Can you work these out from the model? Positions are in its coordinate system, mm. A direction names the side the tool comes from. Give positions to 0.01 mm unless a question says otherwise; leave off trailing zeros. Order: outer loops, then holes, each group sorted by start corner. A loop starts at its lowest first (then second) coordinate and runs counter-clockwise, first axis right, second up. Notation, with made-up numbers: M 51.25,15.5 L 73.25,15.5 A10 cw 73.25,25.5 Z; hole C 80,-5 d4. An arc over 180 degrees is marked long. One line per question, with ' | ' between items. Start each with the question number.
1) Thinking about a two-plate mould opening in X: for faces 1 (the cylindrical face through (-2.343, 17.847, 0.182)), 2 (the cylindrical face through (0.1, -3.1, 0.2)), 3 (the flat face through (0, -4, 13)), which applies, +X half, -X half, draft (parallel to the pull), parting line (faces both ways), or undercut?
2) If we section it at C-C, the plane z = 7.25: Please give me the cut outline in (x, y).
3) If we section it at B-B, the plane x = 0: Please give me the cut outline in (y, z), plus the area to 3 significant figures.
4) If we section it at A-A, the plane y = 0: Please give me the cut outline in (x, z).
5) Please list where these lines run through material, in increasing order: line 1 along Y through (x, z) = (0, -7.5); line 2 along X through (y, z) = (3.5, -6.25); line 3 along X through (y, z) = (13, 0). Write a range as [from, to].
6) If we section it at D-D, the plane y = 14: Please give me the cut outline in (x, z).
7) For faces 4 (the flat face through (-1, 3.5, 0.2)), 5 (the flat face through (0, -4, -13)), which set-ups out of +Z, -Z, +X, -X, +Y, -Y let a thin tool reach every point of the face, with its end or its side?
8) I'm going to push flat-ended pins straight in: pin 1 Ø1.2 at (y, z) = (3.5, -5.5) entering from +X; pin 2 Ø2 at (x, y) = (0, 14) entering from -Z; pin 3 Ø1.5 at (y, z) = (14, 1) entering from -X; pin 4 Ø1.2 at (y, z) = (3.5, 1) entering from -X. Where does each tip first touch, or does it pass through?
```python
from build123d import *

# Parameters (mm, degrees)
SKETCH_1_R      = 18
SKETCH_1_R_2    = 1.25
EXTRUDE_1_DEPTH = 13


with BuildPart() as part:
    # 草图1 → 凸台-拉伸1 (new, symmetric)
    with BuildSketch(Plane.XY):
        Circle(SKETCH_1_R)
        with Locations((0, 14)):
            Circle(SKETCH_1_R_2, mode=Mode.SUBTRACT)
        with BuildLine():
            Line((-1, 2.93428015), (-1, 4))
            Line((-1, 4), (1, 4))
            Line((1, 4), (1, 2.93428015))
            ThreePointArc((1, 2.93428015), (0, -3.1), (-1, 2.93428015))
        make_face(mode=Mode.SUBTRACT)
    extrude(amount=EXTRUDE_1_DEPTH, both=True)


solid = part.part
```
Results found:
1) face 1: parting line | face 2: undercut | face 3: draft
2) outline: C 0,0 d36; hole C 0,14 d2.5; hole M -1,2.93 A3.1 ccw long 1,2.93 L 1,4 L -1,4 Z
3) outline: M -18,-13 L -3.1,-13 L -3.1,13 L -18,13 Z; M 4,-13 L 12.75,-13 L 12.75,13 L 4,13 Z; M 15.25,-13 L 18,-13 L 18,13 L 15.25,13 Z | area: 686 mm²
4) outline: M -18,-13 L -3.1,-13 L -3.1,13 L -18,13 Z; M 3.1,-13 L 18,-13 L 18,13 L 3.1,13 Z
5) line 1: y = [-18, -3.1], [4, 12.75], [15.25, 18] | line 2: x = [-17.66, -1], [1, 17.66] | line 3: x = [-12.45, -0.75], [0.75, 12.45]
6) outline: M -11.31,-13 L -1.25,-13 L -1.25,13 L -11.31,13 Z; M 1.25,-13 L 11.31,-13 L 11.31,13 L 1.25,13 Z
7) face 4: +Z, -Z | face 5: -Z, +X, -X, +Y, -Y
8) pin 1: stops at x = 17.76 | pin 2: passes through | pin 3: stops at x = -12.18 | pin 4: stops at x = -17.76
